Part print with two shaded views. Sizes in mm from the minimum x, y, z corner. Give positions to 0.01 mm unless a question says otherwise; leave off trailing zeros. Write each loop counter-clockwise with the first axis right and the second up, starting at its lowest first coordinate (ties: lowest second). Pieces come first, ordered by that corner, then holes. Notation, with made-up numbers: (23.5, -27.75) -> (60.5, -27.75) arc R23 ccw to (60.5, 10.25) -> close; hole circle Ø6 at (59, 71). An arc over 180 degrees is marked (long way). Write item = value, one per line. Start each with the question number.
Q1. Saw through at C-C, the plane z = 207. List the corners of the cut face in (x, y), then the cut area to 4 significant figures.
Q2. Mould opens along X. For the marked faces 1 and 2 say: pulls with the +X half, pulls with the -X half, needs draft (parallel to the pull), parting line crosses it, or undercut.
Q3. Saw through at A-A, the plane z = 139. List the corners of the cut face in (x, y).
Q4. Drop a flat-ended pin along its axis: P1, Ø12, axis at x = 12.5, z = 77, coming from the +Y side. Give the stop position or say it passes through.
Q5. Saw through at B-B, the plane x = 17. List the corners of the cut face in (y, z), then the cut area to 3 significant figures.
Q6. Wall check: line 1 (X direction, y = 7.75, z = 83); line 2 (X direction, y = 1.5, z = 126); line 3 (Y direction, x = 14, z = 180). Give the ranges that are in metal, low to high.
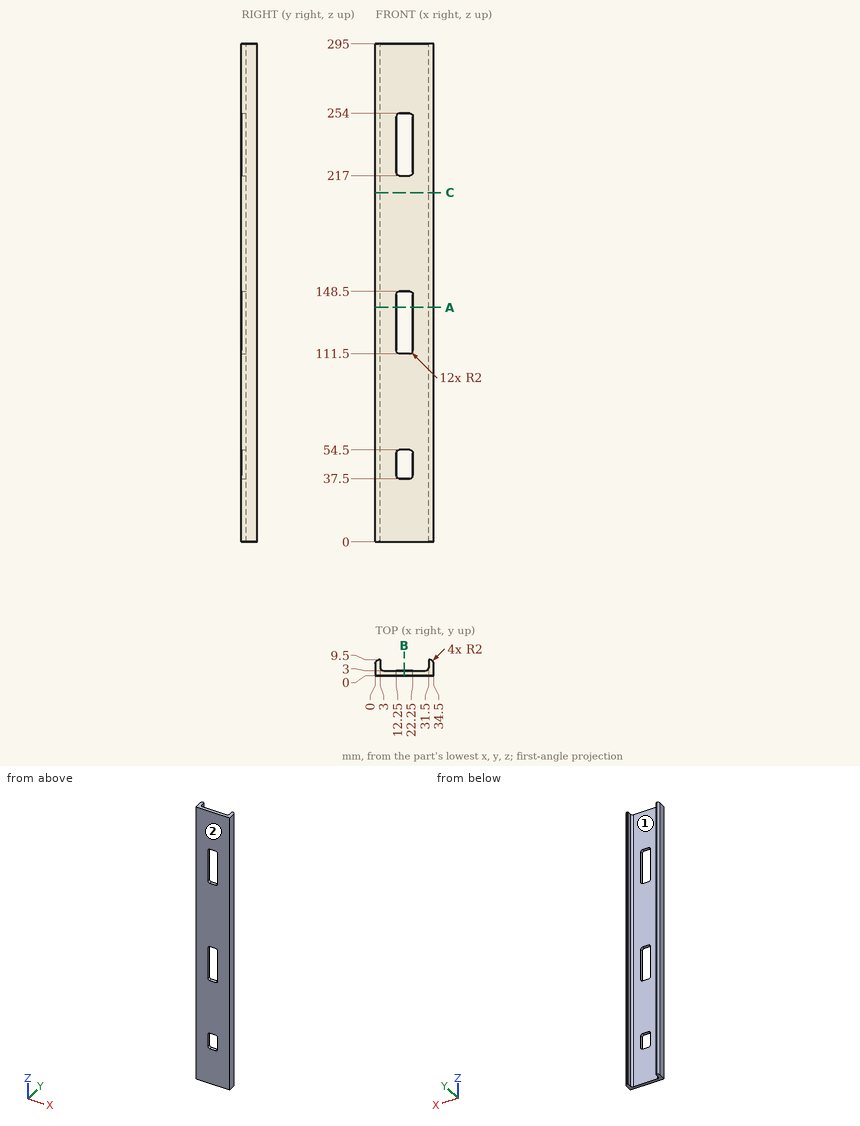
Report:
q1.outline = (0, 0) -> (34.5, 0) -> (34.5, 7.5) arc R2 ccw to (32.5, 9.5) -> (31.5, 9.5) -> (31.5, 5) arc R2 cw to (29.5, 3) -> (5, 3) arc R2 cw to (3, 5) -> (3, 9.5) -> (2, 9.5) arc R2 ccw to (0, 7.5) -> close
q1.area = 142.5 mm2
q2.face_1 = undercut
q2.face_2 = needs draft
q3.outline = (0, 0) -> (12.25, 0) -> (12.25, 3) -> (5, 3) arc R2 cw to (3, 5) -> (3, 9.5) -> (2, 9.5) arc R2 ccw to (0, 7.5) -> close; (22.25, 0) -> (34.5, 0) -> (34.5, 7.5) arc R2 ccw to (32.5, 9.5) -> (31.5, 9.5) -> (31.5, 5) arc R2 cw to (29.5, 3) -> (22.25, 3) -> close
q4.P1 = 3
q5.outline = (0, 0) -> (3, 0) -> (3, 37.5) -> (0, 37.5) -> close; (0, 54.5) -> (3, 54.5) -> (3, 111.5) -> (0, 111.5) -> close; (0, 148.5) -> (3, 148.5) -> (3, 217) -> (0, 217) -> close; (0, 254) -> (3, 254) -> (3, 295) -> (0, 295) -> close
q5.area = 612 mm2
q6.line_1 = 0.02 to 3, 31.5 to 34.48
q6.line_2 = 0 to 12.25, 22.25 to 34.5
q6.line_3 = 0 to 3
